from build123d import *

# Parameters (mm, degrees)
BOSS_EXTRUDE7_DEPTH = 11


with BuildPart() as part:
    # Sketch2 → Boss-Extrude7 (new body)
    with BuildSketch(Plane.XY):
        with BuildLine():
            Line((-0.187241808, 0), (-0.187241808, 98))
            ThreePointArc((-0.187241808, 98), (0.39854463, 99.414213562), (1.812758192, 100))
            Line((1.812758192, 100), (51.812758192, 100))
            ThreePointArc((51.812758192, 100), (53.226971755, 99.414213562), (53.812758192, 98))
            Line((53.812758192, 98), (53.812758192, 55))
            ThreePointArc((53.812758192, 55), (56.335532617, 49.169048105), (62.312758192, 47.015640289))
            ThreePointArc((62.312758192, 47.015640289), (68.289983767, 49.169048105), (70.812758192, 55))
            Line((70.812758192, 55), (70.812758192, 98))
            ThreePointArc((70.812758192, 98), (71.39854463, 99.414213562), (72.812758192, 100))
            Line((72.812758192, 100), (122.812758192, 100))
            ThreePointArc((122.812758192, 100), (124.226971755, 99.414213562), (124.812758192, 98))
            Line((124.812758192, 98), (124.812758192, 0))
            Line((124.812758192, 0), (100.112758192, 0))
            Line((100.112758192, 0), (100.112758192, 11))
            Line((100.112758192, 11), (74.662758192, 11))
            Line((74.662758192, 11), (74.662758192, 0))
            Line((74.662758192, 0), (49.962758192, 0))
            Line((49.962758192, 0), (49.962758192, 11))
            Line((49.962758192, 11), (24.512758192, 11))
            Line((24.512758192, 11), (24.512758192, 0))
            Line((24.512758192, 0), (-0.187241808, 0))
        make_face()
        with BuildLine():
            Line((41.562758192, 69.5), (41.562758192, 84.5))
            ThreePointArc((41.562758192, 84.5), (44.062758192, 87), (46.562758192, 84.5))
            Line((46.562758192, 84.5), (46.562758192, 69.5))
            ThreePointArc((46.562758192, 69.5), (44.062758192, 67), (41.562758192, 69.5))
        make_face(mode=Mode.SUBTRACT)
        with BuildLine():
            Line((83.062758192, 69.5), (83.062758192, 84.5))
            ThreePointArc((83.062758192, 84.5), (80.562758192, 87), (78.062758192, 84.5))
            Line((78.062758192, 84.5), (78.062758192, 69.5))
            ThreePointArc((78.062758192, 69.5), (80.562758192, 67), (83.062758192, 69.5))
        make_face(mode=Mode.SUBTRACT)
        with BuildLine():
            Line((7.462758192, 69.5), (7.462758192, 84.5))
            ThreePointArc((7.462758192, 84.5), (9.312758192, 86.35), (11.162758192, 84.5))
            Line((11.162758192, 84.5), (11.162758192, 69.5))
            ThreePointArc((11.162758192, 69.5), (9.312758192, 67.65), (7.462758192, 69.5))
        make_face(mode=Mode.SUBTRACT)
        with BuildLine():
            Line((22.986098789, 32.023340597), (22.986098789, 47.023340597))
            ThreePointArc((22.986098789, 47.023340597), (24.836098789, 48.873340597), (26.686098789, 47.023340597))
            Line((26.686098789, 47.023340597), (26.686098789, 32.023340597))
            ThreePointArc((26.686098789, 32.023340597), (24.836098789, 30.173340597), (22.986098789, 32.023340597))
        make_face(mode=Mode.SUBTRACT)
        with BuildLine():
            Line((60.462758192, 16.5), (60.462758192, 31.5))
            ThreePointArc((60.462758192, 31.5), (62.312758192, 33.35), (64.162758192, 31.5))
            Line((64.162758192, 31.5), (64.162758192, 16.5))
            ThreePointArc((64.162758192, 16.5), (62.312758192, 14.65), (60.462758192, 16.5))
        make_face(mode=Mode.SUBTRACT)
        with BuildLine():
            Line((97.939417595, 32.023340597), (97.939417595, 47.023340597))
            ThreePointArc((97.939417595, 47.023340597), (99.789417595, 48.873340597), (101.639417595, 47.023340597))
            Line((101.639417595, 47.023340597), (101.639417595, 32.023340597))
            ThreePointArc((101.639417595, 32.023340597), (99.789417595, 30.173340597), (97.939417595, 32.023340597))
        make_face(mode=Mode.SUBTRACT)
        with BuildLine():
            Line((113.462758192, 69.5), (113.462758192, 84.5))
            ThreePointArc((113.462758192, 84.5), (115.312758192, 86.35), (117.162758192, 84.5))
            Line((117.162758192, 84.5), (117.162758192, 69.5))
            ThreePointArc((117.162758192, 69.5), (115.312758192, 67.65), (113.462758192, 69.5))
        make_face(mode=Mode.SUBTRACT)
    extrude(amount=BOSS_EXTRUDE7_DEPTH)


solid = part.part
CAD build for the part. Positions are in the model's coordinates, mm. A direction names the side the tool comes from. Give positions to 0.01 mm unless a question says otherwise; leave off trailing zeros. Loops run counter-clockwise (first coordinate to the right, second up) from the corner with the lowest first, then second, coordinate; pieces in that order, holes last. Notation, with made-up numbers: M 65,47 L 88,47 A29 ccw 88,72 Z; hole C 19,26.5 d2. An arc over 180 degrees is marked long. Write each question's results on one line, items separated by ' | '.
Q1. Band-saw the part on C-C on x = 68.5. Write the cut outline in (y, z), and give its area (3 significant figures).
Geometry check:
outline: M 0,0 L 49.37,0 L 49.37,11 L 0,11 Z | area: 543 mm²
Q2. Band-saw the part on B-B on z = 8.75. Give the number of separate pieces and of enclosed holes in the cut face, and give its area (3 significant figures).
Geometry check:
separate pieces: 1 | enclosed holes: 7 | area: 10,500 mm²
Q3. Probe probe 1 along X at (y, z) = (64, 1.5); probe 2 along X at (y, z) = (23.5, 5); probe 3 along X at (y, z) = (83.5, 1.5). List the from-to ranges inside material, lowest first.
Geometry check:
probe 1: x = -0.19 to 53.81, 70.81 to 124.81 | probe 2: x = -0.19 to 60.46, 64.16 to 124.81 | probe 3: x = -0.19 to 7.46, 11.16 to 41.56, 46.56 to 53.81, 70.81 to 78.06, 83.06 to 113.46, 117.16 to 124.81
Q4. Mould opens along X. For faces 4 (the face through (24.513, 6, 5)), 5 (the face through (-0.187, 48, 5)) say: pulls with the +X half, pulls with the -X half, needs draft (parallel to the pull), parting line crosses it, or undercut.
Geometry check:
face 4: undercut | face 5: pulls with the -X half
Q5. Flat gauge pin, fed straight in: P1, Ø5.5, axis at x = 35.5, z = 4, coming from the -Y side. Where does the tip first touch, or does it go through?
Geometry check:
P1: stops at y = 11
Q6. Which spindle directions (+Z, -Z, +X, -X, +Y, -Y) get a long thin tool onto all of the face, cutting with end or side? Do faces 1 (the face through (115.27, 86.35, 5.42)), 2 (the face through (100.113, 5, 5)), 3 (the face through (70.813, 76, 5)). Say none if no direction does.
Geometry check:
face 1: +Z, -Z | face 2: +Z, -Z, -Y | face 3: +Z, -Z, +Y
Q7. Band-saw the part on A-A on y = 35. Write the cut outline in (x, z), and give its area (3 significant figures).
Geometry check:
outline: M -0.19,0 L 22.99,0 L 22.99,11 L -0.19,11 Z; M 26.69,0 L 97.94,0 L 97.94,11 L 26.69,11 Z; M 101.64,0 L 124.81,0 L 124.81,11 L 101.64,11 Z | area: 1,290 mm²
